Build history of the part. All positions in model axes, mm. A direction names the side the tool comes from. Round coordinates to 2 decimals unless told otherwise and drop trailing zeros. Write each loop counter-clockwise with the first axis right and the second up, starting at its lowest first coordinate (ties: lowest second). Pieces come first, ordered by that corner, then holes.
from build123d import *

# Parameters (mm, degrees)
SKETCH2_R           = 3.175
BOSS_EXTRUDE1_DEPTH = 42.25
CHAMFER1_SIZE       = 0.5


with BuildPart() as part:
    # Sketch2 → Boss-Extrude1 (new body)
    with BuildSketch(Plane.XY):
        Circle(SKETCH2_R)
    extrude(amount=BOSS_EXTRUDE1_DEPTH)

    # Sketch5 → Cut-Revolve1 (revolve, cut)
    with BuildSketch(Plane(origin=(0, 0, 0), x_dir=(0, 0, -1), z_dir=(1, 0, 0)), mode=Mode.PRIVATE) as cut_revolve1_sk:
        with BuildLine():
            Line((-21.25, 3.175), (0, 3.175))
            Line((0, 3.175), (0, 2.38125))
            Line((0, 2.38125), (-19, 2.38125))
            ThreePointArc((-19, 2.38125), (-20.192952122, 2.585504811), (-21.25, 3.175))
        make_face()
    revolve(cut_revolve1_sk.sketch.rotate(Axis((0, 0, 21.25), (0, 0, -1)), 90), axis=Axis((0, 0, 21.25), (0, 0, -1)), mode=Mode.SUBTRACT)

    # Chamfer1
    chamfer1_edges = [part.edges().sort_by_distance(p)[0] for p in [
        (-3.175, 0, 42.25),
        (-2.38125, 0, 0),
    ]]
    chamfer(chamfer1_edges, length=CHAMFER1_SIZE)


solid = part.part
1) Slice it at A-A (y = 0). Write the cut outline in (x, z) (3 decimals).
Results:
outline: (-3.175, 21.25) arc R3.586 cw to (-2.381, 19) - (-2.381, 0.5) - (-1.881, 0) - (1.881, 0) - (2.381, 0.5) - (2.381, 19) arc R3.586 cw to (3.175, 21.25) - (3.175, 41.75) - (2.675, 42.25) - (-2.675, 42.25) - (-3.175, 41.75) - close
2) Which spindle directions (+Z, -Z, +X, -X, +Y, -Y) get a long thin tool onto all of the face, cutting with end or side? Do faces 1 (the cylindrical face through (-0.516, 2.325, 9.88)), 2 (the flat face through (0, 0, 0)). Say none if no direction does.
Results:
face 1: -Z
face 2: -Z, +X, -X, +Y, -Y
3) Pin check, flat tip, straight feed: pin 1 Ø1.5 at (y, z) = (0.5, 6.5) entering from -X. Stop position of the tip, or through.
Results:
pin 1: stops at x = -2.38
4) Slice it at D-D (z = 17). Write the cut outline in (x, y), plus the area to 3 significant figures.
Results:
outline: circle Ø4.76 at (0, 0)
area: 17.8 mm2
5) Wall check: L1, parallel to X at y = 2.25, z = 32.5; L2, parallel to X at y = 0.5, z = 8.5; L3, parallel to Y at x = -1.25, z = 15. Give the ranges that are in metal, low to high.
Results:
L1: x = -2.24 to 2.24
L2: x = -2.33 to 2.33
L3: y = -2.03 to 2.03
6) Slice it at C-C (z = 34). Write the cut outline in (x, y) (3 decimals), plus the area to 3 significant figures.
Results:
outline: circle Ø6.35 at (0, 0)
area: 31.7 mm2
